The drawing under review shows one solid part. Ordinate dimensions are in mm from its lowest x, y, z. A direction names the side the tool comes from. Coordinates: 2 decimals unless noted, no trailing zeros. Order: outer loops, then holes, each group sorted by start corner. A loop starts at its lowest first (then second) coordinate and runs counter-clockwise, first axis right, second up. Notation, with made-up numbers: (-30, -17.75) - (19, -17.75) arc R29 cw to (19, 21.25) - close; hole circle Ø5 at (57.25, 89.5). An arc over 180 degrees is marked (long way). Write each question's results on one line, items separated by ' | '. Start each with the question number.
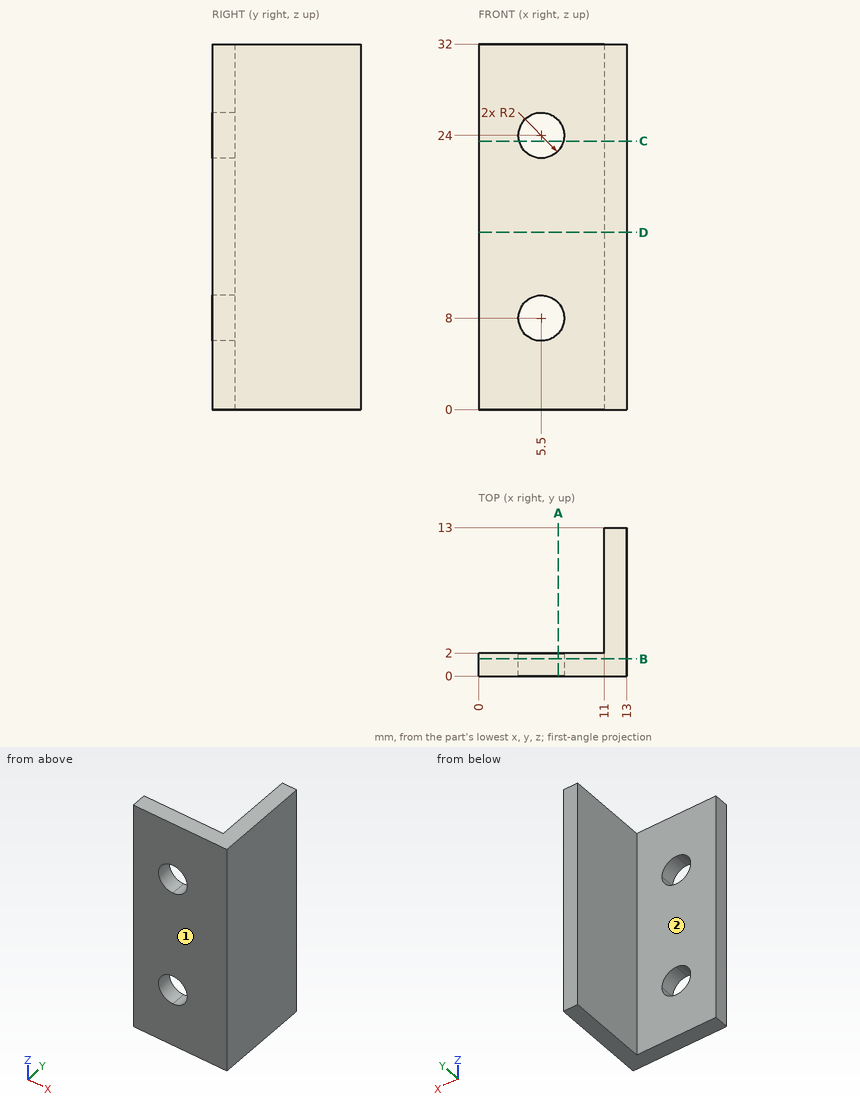
(1) To check wall thickness, follow line 1 along X through (y, z) = (3.5, 3); line 2 along Y through (x, z) = (4.25, 29.5); line 3 along X through (y, z) = (1.5, 7). State the ranges of each line that lie inside material, in increasing order. Write a range as [from, to].
(2) Take a section at C-C (z = 23.5). State the section outline as (x, y) points.
(3) Take a section at B-B (y = 1.5). State the section outline as (x, z) points, plus the area to 3 significant figures.
(4) Take a section at A-A (x = 7). State the section outline as (y, z) points.
(5) Take a section at D-D (z = 15.5). State the section outline as (x, y) points, plus the area to 3 significant figures.
(6) Clearance check with a flat-ended pin moving along its axis: pin 1 (3.5 mm diameter, centred on y = 5, z = 12.5, fed in from -X). State where the tip first meets the part, or that it passes through.
(7) Tool access review of the marked faces 1 and 2: name each direction out of +Z, -Z, +X, -X, +Y, -Y from which nothing blocks a thin tool from reaching the whole face with its end or side.
Worked out:
1) line 1: [11, 13] | line 2: [0, 2] | line 3: [0, 3.77], [7.23, 13]
2) outline: (0, 0) - (3.56, 0) - (3.56, 2) - (0, 2) - close; (7.44, 0) - (13, 0) - (13, 13) - (11, 13) - (11, 2) - (7.44, 2) - close
3) outline: (0, 0) - (13, 0) - (13, 32) - (0, 32) - close; hole circle Ø4 at (5.5, 8); hole circle Ø4 at (5.5, 24) | area: 391 mm^2
4) outline: (0, 0) - (2, 0) - (2, 6.68) - (0, 6.68) - close; (0, 9.32) - (2, 9.32) - (2, 22.68) - (0, 22.68) - close; (0, 25.32) - (2, 25.32) - (2, 32) - (0, 32) - close
5) outline: (0, 0) - (13, 0) - (13, 13) - (11, 13) - (11, 2) - (0, 2) - close | area: 48.0 mm^2
6) pin 1: x = 11
7) face 1: +Z, -Z, +X, -X, -Y | face 2: +Z, -Z, -X, +Y
